Part model, mm, in its own coordinate system. A direction names the side the tool comes from. Round coordinates to 2 decimals unless told otherwise and drop trailing zeros. Loops run counter-clockwise (first coordinate to the right, second up) from the corner with the lowest first, then second, coordinate; pieces in that order, holes last.
1) Band-saw the part on B-B, the plane y = 0. Write the cut outline in (x, z), then the cut area to 3 significant figures.
2) Probe line 1 (Z direction, x = 50, y = -12.5); line 2 (Y direction, x = -23, z = 129.5); line 3 (X direction, y = -4.5, z = 100). List the from-to ranges inside material, lowest first.
3) Band-saw the part on C-C, the plane z = 118. Write the cut outline in (x, y).
4) Band-saw the part on D-D, the plane x = 36.5. Write the cut outline in (y, z), then the cut area to 3 significant figures.
5) 3-axis set-ups, long thin cutter, end or side, ignore diameter. For faces 1 (the flat face through (-1, 0, -10.552)), 2 (the cylindrical face through (-22.638, -17.358, 75.133)): which of +Z, -Z, +X, -X, +Y, -Y reach the whole face in a straight line?
6) Drop flat-ended pins along their axis: P1, Ø5, axis at y = 2, z = 118.5, coming from the -X side; P2, Ø4, axis at y = 14, z = 74, coming from the +X side; P3, Ø1.5, axis at x = 27, z = 15.5, coming from the +Y side. Give the stop position or say it passes through.
7) Band-saw the part on A-A, the plane x = 0. Write the cut outline in (y, z).
from build123d import *

# Parameters (mm, degrees)
F0_R     = 28.526815
F1_DEPTH = 152.4
F2_W     = 122.707962
F2_H     = 62.613734
F3_DEPTH = 10.551801


with BuildPart() as f1:
    # F0 (on Top) → F1 (new body)
    with BuildSketch(Plane.XY):
        Circle(F0_R)
    extrude(amount=F1_DEPTH)

    # F2 (on Top) → F3 (join)
    with BuildSketch(Plane.XY):
        Rectangle(F2_W, F2_H)
    extrude(amount=-F3_DEPTH)


solid = f1.part
Reported:
1. outline: (-61.35, -10.55) - (61.35, -10.55) - (61.35, 0) - (28.53, 0) - (28.53, 152.4) - (-28.53, 152.4) - (-28.53, 0) - (-61.35, 0) - close
1. area: 9,990 mm2
2. line 1: z = -10.55 to 0
2. line 2: y = -16.88 to 16.88
2. line 3: x = -28.17 to 28.17
3. outline: circle Ø57.05 at (0, 0)
4. outline: (-31.31, -10.55) - (31.31, -10.55) - (31.31, 0) - (-31.31, 0) - close
4. area: 661 mm2
5. face 1: -Z, +X, -X, +Y, -Y
5. face 2: +Z
6. P1: stops at x = -28.53
6. P2: stops at x = 25.88
6. P3: stops at y = 11.17
7. outline: (-31.31, -10.55) - (31.31, -10.55) - (31.31, 0) - (28.53, 0) - (28.53, 152.4) - (-28.53, 152.4) - (-28.53, 0) - (-31.31, 0) - close
